```python
from build123d import *

# Parameters (mm, degrees)
ESQUISSE1_R        = 1.5
BOSS_EXTRU_1_DEPTH = 1


with BuildPart() as part:
    # Esquisse1 → Boss.-Extru.1 (new body)
    with BuildSketch(Plane.XY):
        with BuildLine():
            Line((0, 0), (20, 0))
            Line((20, 0), (20, 10))
            Line((20, 10), (14.145081595, 10))
            ThreePointArc((14.145081595, 10), (12.846043489, 10.75), (12.846043489, 12.25))
            Line((12.846043489, 12.25), (20.553669583, 25.6))
            Line((20.553669583, 25.6), (11.893415545, 30.6))
            Line((11.893415545, 30.6), (0, 10))
            Line((0, 10), (0, 0))
        make_face()
        with Locations((5, 5)):
            Circle(ESQUISSE1_R, mode=Mode.SUBTRACT)
        with Locations((15, 5)):
            Circle(ESQUISSE1_R, mode=Mode.SUBTRACT)
        with Locations((13.723542564, 23.769872981)):
            Circle(ESQUISSE1_R, mode=Mode.SUBTRACT)
        with Locations((8.723542564, 15.109618943)):
            Circle(ESQUISSE1_R, mode=Mode.SUBTRACT)
    extrude(amount=BOSS_EXTRU_1_DEPTH)


solid = part.part
```
Could you check a few things on this model? Use its own coordinates, in mm. A direction names the side the tool comes from. Give positions to 0.01 mm unless a question says otherwise; leave off trailing zeros. Loops run counter-clockwise (first coordinate to the right, second up) from the corner with the lowest first, then second, coordinate; pieces in that order, holes last. Notation, with made-up numbers: (44.25, 9) - (86.25, 9) arc R21 cw to (86.25, 15) - close; hole circle Ø2 at (-4.75, 52). An arc over 180 degrees is marked (long way). Answer in a Markdown table with one row per item. Add a question column.
Q1. If we section it at D-D (z = 0.5): List the corners of the cut face in (x, y) for me, plus the area to 3 significant figures.
Q2. We'd pull the mould along X, two halves only. Please class faces 1 (the face through (0, 5.1, 0.5)), 2 (the face through (13.5, 5.07, 0.49)), 3 (the face through (20, 4.9, 0.5)), 4 (the face through (17.1, 10, 0.5)): +X half, -X half, draft (parallel to the pull), parting line (faces both ways), or undercut.
Q3. For pin 1 (10 mm diameter, centred on x = 17, y = 23, fed in from -Z); pin 2 (1.8 mm diameter, centred on x = 8.72, y = 15.11, fed in from +Z), each with a flat end and sliding along its axis, tell me the tip position at first contact or that it passes through.
Q4. If we section it at B-B (x = 14.5): List the corners of the cut face in (y, z) for me, plus the area to 3 significant figures.
Q5. If we section it at A-A (y = 5): List the corners of the cut face in (x, z) for me.
Q6. Please list where these lines run through material, in increasing order: L1, parallel to Y at x = 14, z = 0.1; L2, parallel to X at y = 8, z = 0.4; L3, parallel to Y at x = 15, z = 0.75. Write a range as from..to.
Q7. Which directions (+Z, -Z, +X, -X, +Y, -Y) give clear straight access to the entire face, cutting with the end or side of a thin tool? Please do faces 5 (the face through (9.9, 0, 0.5)), 6 (the face through (16.646, 18.832, 0.493)).
Q8. If we section it at C-C (x = 5): List the corners of the cut face in (y, z) for me, plus the area to 3 significant figures.
The answers:
| question | item | result |
|---|---|---|
| 1 | outline | (0, 0) - (20, 0) - (20, 10) - (14.15, 10) arc R1.5 cw to (12.85, 12.25) - (20.55, 25.6) - (11.89, 30.6) - (0, 10) - close; hole circle Ø3 at (5, 5); hole circle Ø3 at (8.72, 15.11); hole circle Ø3 at (13.72, 23.77); hole circle Ø3 at (15, 5) |
| 1 | area | 382 mm^2 |
| 2 | face 1 | -X half |
| 2 | face 2 | undercut |
| 2 | face 3 | +X half |
| 2 | face 4 | draft |
| 3 | pin 1 | stops at z = 0 |
| 3 | pin 2 | passes through |
| 4 | outline | (0, 0) - (3.59, 0) - (3.59, 1) - (0, 1) - close; (6.41, 0) - (10, 0) - (10, 1) - (6.41, 1) - close; (15.11, 0) - (22.49, 0) - (22.49, 1) - (15.11, 1) - close; (25.05, 0) - (29.1, 0) - (29.1, 1) - (25.05, 1) - close |
| 4 | area | 18.6 mm^2 |
| 5 | outline | (0, 0) - (3.5, 0) - (3.5, 1) - (0, 1) - close; (6.5, 0) - (13.5, 0) - (13.5, 1) - (6.5, 1) - close; (16.5, 0) - (20, 0) - (20, 1) - (16.5, 1) - close |
| 6 | L1 | y = 0..3.88, 6.12..10.01, 14.25..22.3, 25.24..29.38 |
| 6 | L2 | x = 0..20 |
| 6 | L3 | y = 0..3.5, 6.5..10, 15.98..22.98, 24.56..28.81 |
| 7 | face 5 | +Z, -Z, +X, -X, -Y |
| 7 | face 6 | +Z, -Z, +X |
| 8 | outline | (0, 0) - (3.5, 0) - (3.5, 1) - (0, 1) - close; (6.5, 0) - (18.66, 0) - (18.66, 1) - (6.5, 1) - close |
| 8 | area | 15.7 mm^2 |
